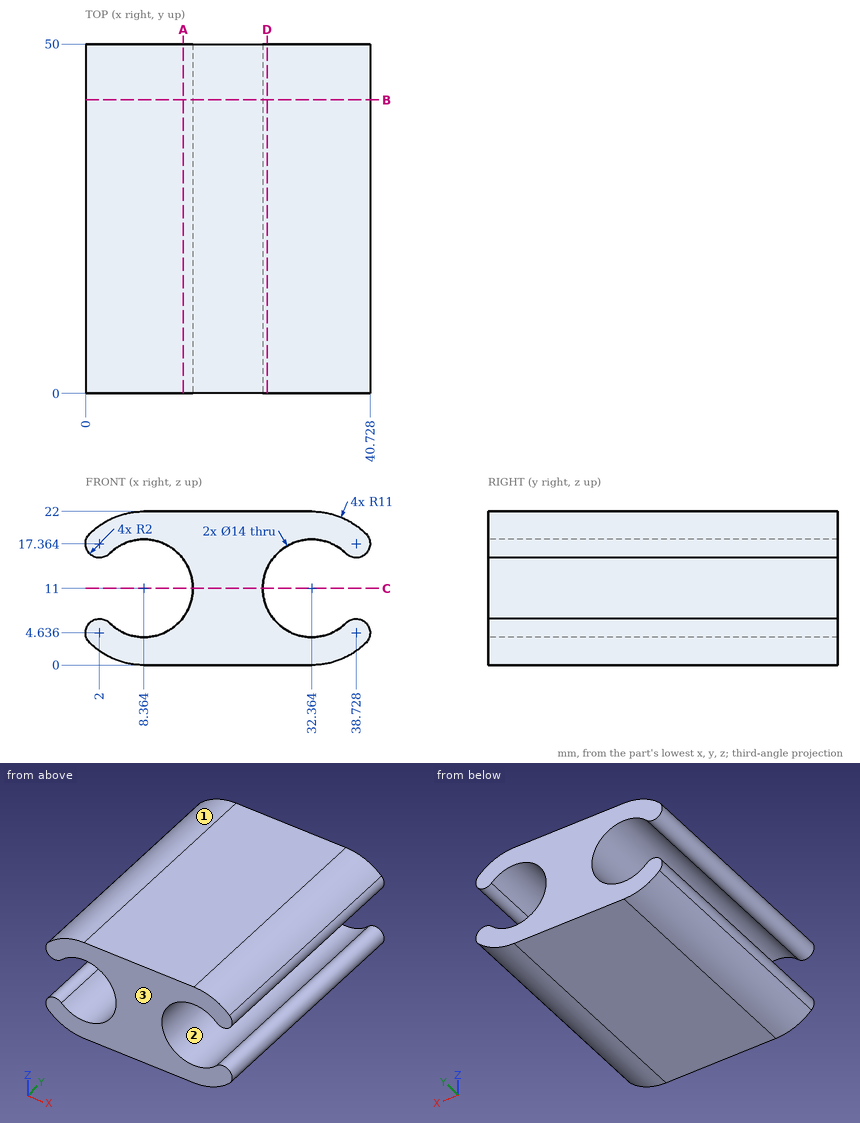
Here's the drawing with two shaded views (mm, measured from the low corner). I have some questions. Round coordinates to 2 decimals unless told otherwise and drop trailing zeros. Write each loop counter-clockwise with the first axis right and the second up, starting at its lowest first coordinate (ties: lowest second). Pieces come first, ordered by that corner, then holes. Notation, with made-up numbers: M 68.25,17 L 72.25,17 A16 cw 72.25,44 Z; hole C -5.5,22.25 d10. An arc over 180 degrees is marked long. Write each question's results on one line, items separated by ' | '. Start each with the question number.
1. Imagine slicing it at D-D on x = 26. List the corners of the cut face in (y, z) for me (1 decimal).
2. I'm going to push flat-ended pins straight in: pin 1 Ø3 at (x, y) = (6, 28.5) entering from +Z; pin 2 Ø5 at (x, y) = (17.5, 32) entering from -Z; pin 3 Ø12.5 at (x, z) = (8.36, 11) entering from -Y. Where does each tip first touch, or does it pass through?
3. I need wall thicknesses on L1, parallel to Z at x = 8, y = 14; L2, parallel to X at y = 10.5, z = 16.75 (1 decimal); L3, parallel to X at y = 24.5, z = 5 (1 decimal). Which ranges of each line are inside material? Lowest first, please. Write a range as from..to.
4. Imagine slicing it at B-B on y = 42. List the corners of the cut face in (x, z) for me, and give its area (3 significant figures).
5. Imagine slicing it at C-C on z = 11. List the corners of the cut face in (x, y) for me, and give its area (3 significant figures).
6. Imagine slicing it at A-A on x = 14. List the corners of the cut face in (y, z) for me.
7. Thinking about a two-plate mould opening in Z: for the marked faces 1, 2 and 3, which applies, +Z half, -Z half, draft (parallel to the pull), parting line (faces both ways), or undercut?
Result sheet:
1) outline: M 0,0 L 50,0 L 50,8.1 L 0,8.1 Z; M 0,13.9 L 50,13.9 L 50,22 L 0,22 Z
2) pin 1: stops at z = 21.97 | pin 2: stops at z = 0 | pin 3: passes through
3) L1: z = 0.01..4.01, 17.99..21.99 | L2: x = 0.1..4.4, 12.4..28.4, 36.4..40.6 | L3: x = 0..4.8, 12..28.8, 36..40.7
4) outline: M 0.59,3.22 A11 ccw 8.36,0 L 32.36,0 A11 ccw 40.14,3.22 A2 ccw 37.31,6.05 A7 cw long 37.31,15.95 A2 ccw 40.14,18.78 A11 ccw 32.36,22 L 8.36,22 A11 ccw 0.59,18.78 A2 ccw 3.41,15.95 A7 cw long 3.41,6.05 A2 ccw Z | area: 512 mm^2
5) outline: M 15.36,0 L 25.36,0 L 25.36,50 L 15.36,50 Z | area: 500 mm^2
6) outline: M 0,0 L 50,0 L 50,6.85 L 0,6.85 Z; M 0,15.15 L 50,15.15 L 50,22 L 0,22 Z
7) face 1: +Z half | face 2: undercut | face 3: draft
